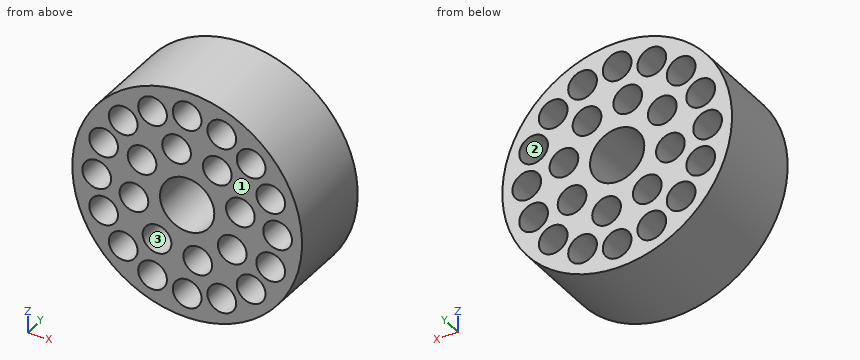
from build123d import *

# Parameters (mm, degrees)
SKETCH1_R           = 6.35
BOSS_EXTRUDE1_DEPTH = 5
SKETCH2_R           = 0.79375
CUT_EXTRUDE1_DEPTH  = 11.278375358
CIRPATTERN1_COUNT   = 16
SKETCH3_R           = 0.79375
CUT_EXTRUDE2_DEPTH  = 11.278375358
CIRPATTERN3_COUNT   = 8
SKETCH4_R           = 1.5
CUT_EXTRUDE3_DEPTH  = 11.278375358


with BuildPart() as part:
    # Sketch1 → Boss-Extrude1 (new body)
    with BuildSketch(Plane(origin=(0, 0, 0), x_dir=(1, 0, 0), z_dir=(0, 1, 0))):
        with Locations(Location((0, 0, 0), (0, 0, 270))):
            Circle(SKETCH1_R)
    extrude(amount=BOSS_EXTRUDE1_DEPTH)

    # Sketch2 → Cut-Extrude1 (cut, through all)
    with BuildSketch(Plane(origin=(0, 5, 0), x_dir=(1, 0, 0), z_dir=(0, 1, 0))):
        with Locations(Location((0, 5, 0), (0, 0, 270))):
            Circle(SKETCH2_R)
    cut_extrude1 = extrude(amount=-CUT_EXTRUDE1_DEPTH, mode=Mode.SUBTRACT)

    # CirPattern1: Cut-Extrude1 ×16 about axis
    cirpattern1_axis = Axis((0, 0, 0), (0, 1, 0))
    for i in range(1, CIRPATTERN1_COUNT):
        add(cut_extrude1.rotate(cirpattern1_axis, i * 360 / CIRPATTERN1_COUNT), mode=Mode.SUBTRACT)

    # Sketch3 → Cut-Extrude2 (cut, through all)
    with BuildSketch(Plane(origin=(0, 5, 0), x_dir=(1, 0, 0), z_dir=(0, 1, 0))):
        with Locations(Location((0.585270966, 2.942355841, 0), (0, 0, 270))):
            Circle(SKETCH3_R)
    cut_extrude2 = extrude(amount=-CUT_EXTRUDE2_DEPTH, mode=Mode.SUBTRACT)

    # CirPattern3: Cut-Extrude2 ×8 about axis
    cirpattern3_axis = Axis((0, 0, 0), (0, 1, 0))
    for i in range(1, CIRPATTERN3_COUNT):
        add(cut_extrude2.rotate(cirpattern3_axis, i * 360 / CIRPATTERN3_COUNT), mode=Mode.SUBTRACT)

    # Sketch4 → Cut-Extrude3 (cut, through all)
    with BuildSketch(Plane(origin=(0, 5, 0), x_dir=(1, 0, 0), z_dir=(0, 1, 0))):
        with Locations(Location((0, 0, 0), (0, 0, 270))):
            Circle(SKETCH4_R)
    extrude(amount=-CUT_EXTRUDE3_DEPTH, mode=Mode.SUBTRACT)


solid = part.part
The listing builds one solid part. Answer for the finished solid, in the listing's coordinates (mm). Face numbers are marked on the shaded views. Round coordinates to 2 decimals unless told otherwise and drop trailing zeros. Loops run counter-clockwise (first coordinate to the right, second up) from the corner with the lowest first, then second, coordinate; pieces in that order, holes last. Notation, with made-up numbers: M 16,-6 L 42,-6 A11 cw 42,11 Z; hole C 50,85.5 d4. An arc over 180 degrees is marked long. Return JSON: item names as keys, results as strings.
Q1. Find section C-C, the plane y = 3.55. State how many separate pieces and enclosed holes the cut face has, plus the area to 3 significant figures.
Results list:
{"separate pieces": "1", "enclosed holes": "25", "area": "72.1 mm2"}
Q2. Find the intervals of material crossed by line 1 along Z through (x, y) = (4, 3.9); line 2 along X through (y, z) = (4.15, 3); line 3 along Z through (x, y) = (2.5, 1.3), in increasing order. Write a range as from..to.
Results list:
{"line 1": "z = -4.93..-4.18, -2.89..-2.41, -1.42..1.42, 2.41..2.89, 4.18..4.93", "line 2": "x = -5.6..-4.12, -2.95..-1.38, 0.21..1.05, 2.28..2.95, 4.12..5.6", "line 3": "z = -5.84..-5.15, -4.08..-2.46, -0.87..-0.07, 1.24..4.08, 5.15..5.84"}
Q3. Find section A-A, the plane z = 0. Determine the outline of the cut face in (x, y).
Results list:
{"outline": "M -6.35,0 L -5.79,0 L -5.79,5 L -6.35,5 Z; M -4.21,0 L -3.48,0 L -3.48,5 L -4.21,5 Z; M -2.41,0 L -1.5,0 L -1.5,5 L -2.41,5 Z; M 1.5,0 L 2.41,0 L 2.41,5 L 1.5,5 Z; M 3.48,0 L 4.21,0 L 4.21,5 L 3.48,5 Z; M 5.79,0 L 6.35,0 L 6.35,5 L 5.79,5 Z"}
Q4. Find section D-D, the plane z = -5. Determine the outline of the cut face in (x, y), plus the area to 3 significant figures.
Results list:
{"outline": "M -3.91,0 L -2.61,0 L -2.61,5 L -3.91,5 Z; M -1.22,0 L -0.79,0 L -0.79,5 L -1.22,5 Z; M 0.79,0 L 1.22,0 L 1.22,5 L 0.79,5 Z; M 2.61,0 L 3.91,0 L 3.91,5 L 2.61,5 Z", "area": "17.3 mm2"}
Q5. Find section B-B, the plane x = -5. Determine the outline of the cut face in (y, z).
Results list:
{"outline": "M 0,-3.91 L 5,-3.91 L 5,-2.61 L 0,-2.61 Z; M 0,-1.22 L 5,-1.22 L 5,-0.79 L 0,-0.79 Z; M 0,0.79 L 5,0.79 L 5,1.22 L 0,1.22 Z; M 0,2.61 L 5,2.61 L 5,3.91 L 0,3.91 Z"}
Q6. The mould has two halves that part along X. Classify the marked faces 1, 2 and 3: released by +X, released by -X, zero draft, split by the parting line, or undercut.
Results list:
{"face 1": "zero draft", "face 2": "undercut", "face 3": "undercut"}
Q7. Each of these flat-tipped pins is pushed along its axis until it touches: pin 1 Ø3 at (x, y) = (1, 4) entering from -Z; pin 2 Ø1 at (x, y) = (-4.5, 3.5) entering from -Z; pin 3 Ø1 at (x, z) = (3.54, 3.54) entering from +Y; pin 4 Ø2 at (y, z) = (2.5, -4) entering from -X. Where does it stop, or does it pass through?
Results list:
{"pin 1": "stops at z = -6.35", "pin 2": "stops at z = -4.93", "pin 3": "passes through", "pin 4": "stops at x = -5.6"}
